Geometry check sheet. Reference: the model listing, model coordinates, mm. Give positions to 0.01 mm unless a question says otherwise; leave off trailing zeros. Loops run counter-clockwise (first coordinate to the right, second up) from the corner with the lowest first, then second, coordinate; pieces in that order, holes last. Notation, with made-up numbers: (-26.75, 41.5) - (1.25, 41.5) arc R6 cw to (1.25, 46.5) - close; hole circle Ø6 at (70.25, 3). An arc over 180 degrees is marked (long way). Use a Markdown table: item, result. Add a question column.
1. Material ranges on L1, parallel to Y at x = -15, z = 1.45; L2, parallel to X at y = -0.5, z = 0.6; L3, parallel to X at y = 3, z = 0.5, recorded low to high.
2. Cross-section at B-B on y = 0. Enter the section's corners in (x, z), and give its area (3 significant figures).
3. Depth check by flat-ended pin: P1, Ø2, axis at x = 9, y = 3, coming from the -Z side. Enter the tip coordinate at first touch or a pass-through.
4. Cross-section at C-C on z = 0.4. Enter the section's corners in (x, y).
5. Cross-section at A-A on x = -15. Enter the section's corners in (y, z), and give its area (4 significant figures).
6. Draft check along X on faces 1 (the cylindrical face through (-16.25, 0.05, 1.27)), 2 (the cylindrical face through (13.75, 0.05, 1.27)), 3 (the cylindrical face through (22, -4, 1)), 4 (the flat face through (0, 0, 0)). Enter one of: pulls with the +X half, pulls with the -X half, needs draft (parallel to the pull), parting line crosses it, or undercut.
from build123d import *

# Parameters (mm, degrees)
F0_W     = 90
F0_H     = 20
F1_DEPTH = 5
F2_R     = 2.5
F3_DEPTH = 5
F4_R     = 5
F5_SCALE = 0.5


with BuildPart() as f1:
    # F0 (on Top) → F1 (new body)
    with BuildSketch(Plane.XY):
        Rectangle(F0_W, F0_H)
    extrude(amount=F1_DEPTH)

    # F2 (on face) → F3 (cut)
    with BuildSketch(Plane.XY.offset(5)):
        with Locations((-30, 0)):
            Circle(F2_R)
        with Locations((30, 0)):
            Circle(F2_R)
    extrude(amount=-F3_DEPTH, mode=Mode.SUBTRACT)

    # F4
    f4_edges = [f1.edges().sort_by_distance(p)[0] for p in [
        (-45, 10, 2.5),
        (-45, -10, 2.5),
        (45, -10, 2.5),
        (45, 10, 2.5),
    ]]
    fillet(f4_edges, radius=F4_R)


with BuildPart() as f1_1:
    # F5: moved
    add(f1.part.scale(F5_SCALE))


solid = f1_1.part
Values found:
| question | item | result |
|---|---|---|
| 1 | L1 | y = -5 to -1.25, 1.25 to 5 |
| 1 | L2 | x = -22.5 to -16.15, -13.85 to 13.85, 16.15 to 22.5 |
| 1 | L3 | x = -22.45 to 22.45 |
| 2 | outline | (-22.5, 0) - (-16.25, 0) - (-16.25, 2.5) - (-22.5, 2.5) - close; (-13.75, 0) - (13.75, 0) - (13.75, 2.5) - (-13.75, 2.5) - close; (16.25, 0) - (22.5, 0) - (22.5, 2.5) - (16.25, 2.5) - close |
| 2 | area | 100 mm2 |
| 3 | P1 | stops at z = 0 |
| 4 | outline | (-22.5, -2.5) arc R2.5 ccw to (-20, -5) - (20, -5) arc R2.5 ccw to (22.5, -2.5) - (22.5, 2.5) arc R2.5 ccw to (20, 5) - (-20, 5) arc R2.5 ccw to (-22.5, 2.5) - close; hole circle Ø2.5 at (-15, 0); hole circle Ø2.5 at (15, 0) |
| 5 | outline | (-5, 0) - (-1.25, 0) - (-1.25, 2.5) - (-5, 2.5) - close; (1.25, 0) - (5, 0) - (5, 2.5) - (1.25, 2.5) - close |
| 5 | area | 18.75 mm2 |
| 6 | face 1 | undercut |
| 6 | face 2 | undercut |
| 6 | face 3 | pulls with the +X half |
| 6 | face 4 | needs draft |
